Part model, mm, in its own coordinate system. Face numbers are marked on the shaded views. A direction names the side the tool comes from. Coordinates: 2 decimals unless noted, no trailing zeros. Write each loop counter-clockwise with the first axis right and the second up, starting at its lowest first coordinate (ties: lowest second). Pieces come first, ordered by that corner, then holes. Notation, with made-up numbers: (86, 39.25) -> (106, 39.25) arc R22 ccw to (106, 76.25) -> close; hole circle Ø11 at (25, 3.5). An arc over 180 degrees is marked (long way). Write item = value, one per line. Start each with the question number.
Q1. Probe line 1 (Y direction, x = 558, z = 135); line 2 (Y direction, x = 171, z = 22); line 3 (Y direction, x = 670, z = 101). List the from-to ranges inside material, lowest first.
Q2. Band-saw the part on B-B, the plane z = 94. List the corners of the cut face in (x, y), plus the area to 3 significant figures.
Q3. Band-saw the part on C-C, the plane y = 29. List the corners of the cut face in (x, z).
Q4. Band-saw the part on A-A, the plane x = 476. List the corners of the cut face in (y, z), plus the area to 3 significant figures.
Q5. Band-saw the part on D-D, the plane y = -117. List the corners of the cut face in (x, z), plus the area to 3 significant figures.
Q6. Tool access for the marked faces 5, 6 and 7: list every direction of +Z, -Z, +X, -X, +Y, -Y with a clear straight run to the whole face (end or side of a thin tool).
Q7. Pin check, flat tips, straight feed: P1, Ø2, axis at y = -198, z = 79.5, coming from the -X side; P2, Ø4.5, axis at x = 748.5, y = -110, coming from the +Z side; P3, Ø3, axis at x = 229, y = 186, coming from the +Z side. Stop position of each tip, or through.
Q8. Pull direction Y, two halves, no side cores. Call the marked faces 1, 2, 3 and 4: released by +Y, released by -Y, zero draft, split by the parting line, or undercut.
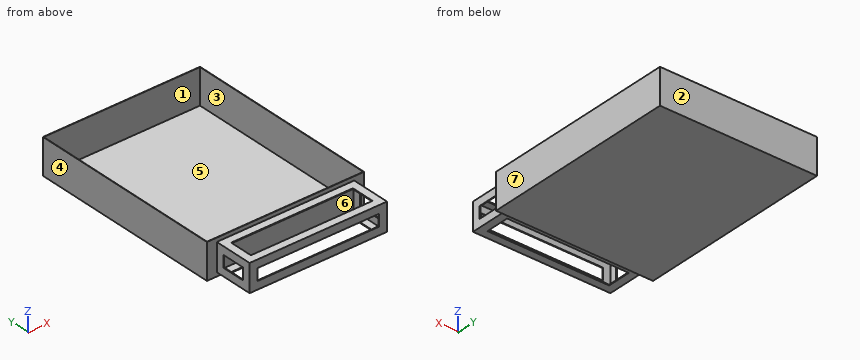
from build123d import *

# Parameters (mm, degrees)
SKETCH_1_W          = 800
SKETCH_1_H          = 1000
EXTRUDE_1_DEPTH     = 180
SHELL_1_T           = -1.8
SKETCH_2_W          = 700
SKETCH_2_H          = 140
SKETCH_2_W_2        = 692
SKETCH_2_H_2        = 132
EXTRUDE_2_DEPTH     = 200
SKETCH_3_W          = 700
SKETCH_3_H          = 140
SKETCH_3_W_2        = 620
SKETCH_3_H_2        = 60
EXTRUDE_3_DEPTH     = 4
SKETCH_4_W          = 620
SKETCH_4_H          = 120
CUT_EXTRUDE_1_DEPTH = 140
SKETCH_5_W          = 60
SKETCH_5_H          = 120
CUT_EXTRUDE_2_DEPTH = 700


with BuildPart() as part:
    # 草图1 → 凸台-拉伸1 (new body)
    with BuildSketch(Plane.XY):
        with Locations((400, 500)):
            Rectangle(SKETCH_1_W, SKETCH_1_H)
    extrude(amount=EXTRUDE_1_DEPTH)

    # 抽壳1
    shell_1_openings = [part.faces().sort_by_distance(p)[0] for p in [
        (400, 500, 180),
    ]]
    offset(amount=SHELL_1_T, openings=shell_1_openings, kind=Kind.INTERSECTION)

    # 草图2 → 凸台-拉伸2 (add)
    with BuildSketch(Plane.XZ):
        with Locations((400, 90)):
            Rectangle(SKETCH_2_W, SKETCH_2_H)
        with Locations((400, 90)):
            Rectangle(SKETCH_2_W_2, SKETCH_2_H_2, mode=Mode.SUBTRACT)
    extrude(amount=EXTRUDE_2_DEPTH)

    # 草图3 → 凸台-拉伸3 (add)
    with BuildSketch(Plane.XZ.offset(200)):
        with Locations((400, 90)):
            Rectangle(SKETCH_3_W, SKETCH_3_H)
        with Locations((400, 90)):
            Rectangle(SKETCH_3_W_2, SKETCH_3_H_2, mode=Mode.SUBTRACT)
    extrude(amount=-EXTRUDE_3_DEPTH)

    # 草图4 → 切除-拉伸1 (cut)
    with BuildSketch(Plane(origin=(0, 0, 20), x_dir=(-1, 0, 0), z_dir=(0, 0, -1))):
        with Locations((-400, -100)):
            Rectangle(SKETCH_4_W, SKETCH_4_H)
    extrude(amount=-CUT_EXTRUDE_1_DEPTH, mode=Mode.SUBTRACT)

    # 草图5 → 切除-拉伸2 (cut)
    with BuildSketch(Plane(origin=(750, 0, 0), x_dir=(0, 0, -1), z_dir=(1, 0, 0))):
        with Locations((-90, -100)):
            Rectangle(SKETCH_5_W, SKETCH_5_H)
    extrude(amount=-CUT_EXTRUDE_2_DEPTH, mode=Mode.SUBTRACT)


solid = part.part
Ans:
q1.line_1 = -200 to -196, 0 to 1.8, 998.2 to 1000
q1.line_2 = -200 to -160, -40 to 1.8, 998.2 to 1000
q1.line_3 = 0 to 1.8, 998.2 to 1000
q2.outline = (0, 0) -> (50, 0) -> (50, -40) -> (54, -40) -> (54, 0) -> (746, 0) -> (746, -40) -> (750, -40) -> (750, 0) -> (800, 0) -> (800, 1000) -> (0, 1000) -> close; (50, -200) -> (90, -200) -> (90, -196) -> (54, -196) -> (54, -160) -> (50, -160) -> close; (710, -200) -> (750, -200) -> (750, -160) -> (746, -160) -> (746, -196) -> (710, -196) -> close; hole (1.8, 1.8) -> (798.2, 1.8) -> (798.2, 998.2) -> (1.8, 998.2) -> close
q2.area = 7,400 mm2
q3.outline = (0, 0) -> (800, 0) -> (800, 180) -> (798.2, 180) -> (798.2, 1.8) -> (1.8, 1.8) -> (1.8, 180) -> (0, 180) -> close
q4.outline = (-200, 20) -> (-160, 20) -> (-160, 24) -> (-196, 24) -> (-196, 60) -> (-200, 60) -> close; (-200, 120) -> (-196, 120) -> (-196, 156) -> (-160, 156) -> (-160, 160) -> (-200, 160) -> close; (-40, 20) -> (0, 20) -> (0, 0) -> (1000, 0) -> (1000, 180) -> (998.2, 180) -> (998.2, 1.8) -> (1.8, 1.8) -> (1.8, 180) -> (0, 180) -> (0, 160) -> (-40, 160) -> (-40, 156) -> (0, 156) -> (0, 24) -> (-40, 24) -> close
q4.area = 3,370 mm2
q5.outline = (50, 20) -> (90, 20) -> (90, 24) -> (54, 24) -> (54, 60) -> (50, 60) -> close; (50, 120) -> (54, 120) -> (54, 156) -> (90, 156) -> (90, 160) -> (50, 160) -> close; (710, 20) -> (750, 20) -> (750, 60) -> (746, 60) -> (746, 24) -> (710, 24) -> close; (710, 156) -> (746, 156) -> (746, 120) -> (750, 120) -> (750, 160) -> (710, 160) -> close
q5.area = 1,220 mm2
q6.face_5 = +Z
q6.face_6 = none
q6.face_7 = +Z, -Z, +X, +Y, -Y
q7.P1 = 50
q7.P2 = 160
q7.P3 = 1.8
q8.face_1 = undercut
q8.face_2 = released by +Y
q8.face_3 = undercut
q8.face_4 = zero draft
